Design review of the part built by this model. Coordinates are the model's own, in mm. Face numbers are marked on the shaded views. A direction names the side the tool comes from. Coordinates: 2 decimals unless noted, no trailing zeros. Loops run counter-clockwise (first coordinate to the right, second up) from the corner with the lowest first, then second, coordinate; pieces in that order, holes last. Notation, with made-up numbers: (21.25, 42.5) -> (46.25, 42.5) arc R18 cw to (46.25, 65.5) -> close; hole circle Ø7 at (70.25, -38). An arc over 180 degrees is marked (long way). Use one line per item in the form item = value. Start each with the question number.
1. For pin 1 (1.5 mm diameter, centred on y = -126.5, z = -20, fed in from +X); pin 2 (11.5 mm diameter, centred on y = -81.5, z = -4.5, fed in from +X); pin 3 (1.5 mm diameter, centred on x = -1.5, z = 17, fed in from +Y), all flat-tipped, find the tip position at first contact; note any pin that passes through.
2. Consider section A-A (y = 57). State the section outline as (x, z) points, then the cut area to 3 significant figures.
3. Consider section B-B (z = -35.5). State the section outline as (x, y) points, then the cut area to 3 significant figures.
4. Consider section D-D (y = -134). State the section outline as (x, z) points.
5. Wall thickness on line 1 (Z direction, x = 41, y = -168); line 2 (Z direction, x = 76, y = -183); line 3 (X direction, y = -60, z = 0.5): over which ranges is each line inside the solid? List them lowest first. Write a range as from..to.
6. Machinability: for the marked faces 1 and 2, which of the approach directions +Z, -Z, +X, -X, +Y, -Y give a long, thin tool a straight path to every point of the face, cutting with its end or side? Answer none if there is none.
from build123d import *

# Parameters (mm, degrees)
F0_W         = 192.698314786
F0_H         = 17.6181327552
F1_DEPTH     = 293.624
F2_SIZE2     = 17.5976362049
F2_SIZE      = 30.48
F3_W         = 155.5479988456
F3_H         = 14.7782256827
F4_DEPTH     = 262.8138
F5_SIZE2     = 23.1696433115
F5_SIZE      = 14.478
F6_W         = 120.3552596271
F6_H         = 14.3881891854
F7_DEPTH     = 239.5982
F8_T4_DEPTH  = 240.1584395307
F9_W         = 77.968429774
F9_H         = 12.2494040988
F10_DEPTH    = 216.408
F11_T4_DEPTH = 168.8399476849
F12_W        = 28.5819442943
F12_H        = 12.4438395724
F13_DEPTH    = 198.628
F14_SIZE2    = 18.2636685711
F14_SIZE     = 12.319
F15_T1_DEPTH = 255.6446994283
F17_DEPTH    = 250.698
F18_DEPTH    = 250.444


# Not quite as in the source:
# - a fillet or chamfer that OpenCascade refuses, or shapes differently, is made with other operations: its cross-section is extruded or revolved along the edge and cut away or added


with BuildPart() as f1:
    # F0 (on Front) → F1 (new body)
    with BuildSketch(Plane.XZ):
        with Locations((2.8250664473, -34.9617386237)):
            Rectangle(F0_W, F0_H)
    extrude(amount=F1_DEPTH)

    # F2
    f2_edges = [f1.edges().sort_by_distance(p)[0] for p in [
        (2.825066, -293.624, -26.152672),
    ]]
    f2_side = f1.faces().sort_by_distance((2.825066, -146.812, -26.152672))[0]
    chamfer(f2_edges, length=F2_SIZE, length2=F2_SIZE2, reference=f2_side)

    # F3 (on face) → F4 (join)
    with BuildSketch(Plane(origin=(0, 0, 0), x_dir=(-1, 0, 0), z_dir=(0, 1, 0))):
        with Locations((-3.2139383256, -18.7635594048)):
            Rectangle(F3_W, F3_H)
    extrude(amount=-F4_DEPTH)

    # F5
    f5_edges = [f1.edges().sort_by_distance(p)[0] for p in [
        (3.213938, -262.8138, -11.374447),
    ]]
    f5_side = f1.faces().sort_by_distance((3.213938, -262.8138, -18.763559))[0]
    chamfer(f5_edges, length=F5_SIZE, length2=F5_SIZE2, reference=f5_side)

    # F6 (on face) → F7 (join)
    with BuildSketch(Plane(origin=(0, 0, 0), x_dir=(-1, 0, 0), z_dir=(0, 1, 0))):
        with Locations((-4.0888953954, -4.1803519707)):
            Rectangle(F6_W, F6_H)
    extrude(amount=-F7_DEPTH)

    # F8: chamfer of 14.478 x 23.1696433115 on 1 edges, made by hand


with BuildPart() as f8_tool2:
    # F8_s3 → F8_t4 (new body)
    with BuildSketch(Plane.YZ.offset(-115.99032437)):
        Polygon((-239.5982, -11.464257378), (-216.4285566885, 3.013742622), (-239.5982, 3.013742622), align=None)
    extrude(amount=F8_T4_DEPTH)

    split(bisect_by=Plane.XY.offset(-11.3744465634), keep=Keep.TOP)


with BuildPart() as f1_1:
    add(f1.part)

    # F8_t1: cut F8_tool2
    add(f8_tool2.part, mode=Mode.SUBTRACT)

    # F9 (on face) → F10 (join)
    with BuildSketch(Plane(origin=(0, 0, 0), x_dir=(-1, 0, 0), z_dir=(0, 1, 0))):
        with Locations((-4.2833294719, 9.1384446714)):
            Rectangle(F9_W, F9_H)
    extrude(amount=-F10_DEPTH)

    # F11: chamfer of 12.319 x 17.5933552951 on 1 edges, made by hand


with BuildPart() as f11_tool2:
    # F11_s3 → F11_t4 (new body)
    with BuildSketch(Plane.YZ.offset(-80.1366443705)):
        Polygon((-216.408, 2.9441467208), (-198.8146447049, 15.2631467208), (-216.408, 15.2631467208), align=None)
    extrude(amount=F11_T4_DEPTH)

    split(bisect_by=Plane.XY.offset(3.013742622), keep=Keep.TOP)


with BuildPart() as f1_2:
    add(f1_1.part)

    # F11_t1: cut F11_tool2
    add(f11_tool2.part, mode=Mode.SUBTRACT)

    # F12 (on face) → F13 (join)
    with BuildSketch(Plane(origin=(0, 0, 0), x_dir=(-1, 0, 0), z_dir=(0, 1, 0))):
        with Locations((-3.5055889748, 21.485066507)):
            Rectangle(F12_W, F12_H)
    extrude(amount=-F13_DEPTH)

    # F14
    f14_edges = [f1_2.edges().sort_by_distance(p)[0] for p in [
        (3.505589, -198.628, 27.706986),
    ]]
    f14_side = f1_2.faces().sort_by_distance((3.505589, -198.628, 21.485067))[0]
    chamfer(f14_edges, length=F14_SIZE, length2=F14_SIZE2, reference=f14_side)

    # F15: fillet of radius 15.3302561211 on 2 edges, made by hand

    # F15_s2 → F15_t1 (cut)
    with BuildSketch(Plane.XZ.offset(-37.6401839997)):
        with BuildLine():
            ThreePointArc((2.7404875221, 27.7069862932), (12.5069415299, 24.1933764328), (17.7965611219, 15.2631467208))
            Line((17.7965611219, 15.2631467208), (17.7965611219, 27.7069862932))
            Line((17.7965611219, 27.7069862932), (2.7404875221, 27.7069862932))
        make_face()
        with BuildLine():
            ThreePointArc((-10.7853831723, 15.2631467208), (-5.4957635803, 24.1933764328), (4.2706904276, 27.7069862932))
            Line((4.2706904276, 27.7069862932), (-10.7853831723, 27.7069862932))
            Line((-10.7853831723, 27.7069862932), (-10.7853831723, 15.2631467208))
        make_face()
    extrude(amount=F15_T1_DEPTH, mode=Mode.SUBTRACT)

    # F16 (on face) → F17 (join)
    with BuildSketch(Plane(origin=(0, 0, 0), x_dir=(-1, 0, 0), z_dir=(0, 1, 0))):
        Polygon((-80.9879377484, -27.7069862932), (-80.9879377484, -43.7708050013), (74.5600610971, -43.7708050013), (74.5600610971, -28.4847263247), (10.7853831723, 15.2631467208), (-17.7965611219, 15.2631467208), align=None)
    extrude(amount=F17_DEPTH)

    # F18 (add): a face of the model
    f18_faces = [f1_2.faces().sort_by_distance(p)[0] for p in [
        (3.5055889748, 0, 20.394937783),
    ]]
    extrude(f18_faces, amount=F18_DEPTH)


solid = f1_2.part
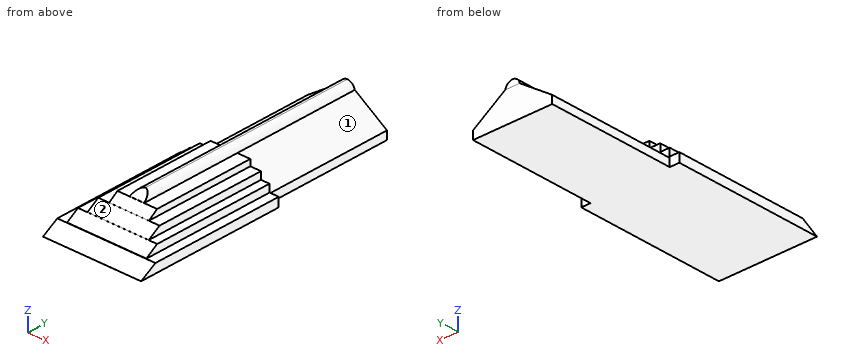
Geometry check:
q1.pin_1 = 80.99
q1.pin_2 = 64.27
q1.pin_3 = 250.44
q2.outline = (-74.56, -43.77) -> (80.99, -43.77) -> (80.99, -27.71) -> (17.8, 15.26) arc R15.33 ccw to (3.51, 27.69) arc R15.33 ccw to (-10.79, 15.26) -> (-74.56, -28.48) -> close
q2.area = 6,690 mm²
q3.outline = (-93.52, -279.33) -> (99.17, -279.33) -> (99.17, 0) -> (80.99, 0) -> (80.99, 250.7) -> (-74.56, 250.7) -> (-74.56, 0) -> (-93.52, 0) -> close
q3.area = 92,800 mm²
q4.outline = (-93.52, -43.77) -> (99.17, -43.77) -> (99.17, -26.15) -> (80.99, -26.15) -> (80.99, -11.37) -> (64.27, -11.37) -> (64.27, 3.01) -> (43.27, 3.01) -> (43.27, 15.26) -> (17.8, 15.26) arc R15.33 ccw to (3.51, 27.69) arc R15.33 ccw to (-10.79, 15.26) -> (-34.7, 15.26) -> (-34.7, 3.01) -> (-56.09, 3.01) -> (-56.09, -11.37) -> (-74.56, -11.37) -> (-74.56, -26.15) -> (-93.52, -26.15) -> close
q5.line_1 = -43.77..15.26
q5.line_2 = -43.77..-11.37
q5.line_3 = -56.09..64.27
q6.face_1 = +Z, +X, +Y
q6.face_2 = +Z, +X, -X, -Y
